Here's how the part is built. I have some questions about the finished solid (model axes, mm). A direction names the side the tool comes from. Round coordinates to 2 decimals unless told otherwise and drop trailing zeros. Order: outer loops, then holes, each group sorted by start corner. A loop starts at its lowest first (then second) coordinate and runs counter-clockwise, first axis right, second up. Notation, with made-up numbers: M -3,-17.5 L 41,-17.5 A18 cw 41,2.5 Z; hole C -7.75,19 d10. An arc over 180 degrees is marked long. Answer as CSV lines item,"result". Start each with the question number.
```python
from build123d import *
from build123d.topology import SkipClean

# Parameters (mm, degrees)
SKETCH1_W           = 25.4
SKETCH1_H           = 25.4
SKETCH1_R           = 1.5
BOSS_EXTRUDE1_DEPTH = 2.54
SKETCH3_W           = 25.4
SKETCH3_H           = 12.7
CUT_EXTRUDE1_DEPTH  = 19.139228208
BOSS_EXTRUDE2_START = 6.35
SKETCH4_R           = 3.175
SKETCH4_R_2         = 1.5
BOSS_EXTRUDE2_DEPTH = 6.35
FILLET1_R           = 6.35


with BuildPart() as part:
    # Sketch1 → Boss-Extrude1 (new body)
    with BuildSketch(Plane(origin=(0, 0, 0), x_dir=(1, 0, 0), z_dir=(0, 1, 0))):
        Rectangle(SKETCH1_W, SKETCH1_H)
        with Locations(Location((-6.35, 6.35, 0), (0, 0, 270))):
            Circle(SKETCH1_R, mode=Mode.SUBTRACT)
        with Locations(Location((6.35, 6.35, 0), (0, 0, 270))):
            Circle(SKETCH1_R, mode=Mode.SUBTRACT)
        with Locations(Location((6.35, -6.35, 0), (0, 0, 270))):
            Circle(SKETCH1_R, mode=Mode.SUBTRACT)
        with Locations(Location((-6.35, -6.35, 0), (0, 0, 270))):
            Circle(SKETCH1_R, mode=Mode.SUBTRACT)
    extrude(amount=BOSS_EXTRUDE1_DEPTH)

    # Sketch3 → Cut-Extrude1 (cut, through all)
    with BuildSketch(Plane.XZ):
        with Locations((0, -6.35)):
            Rectangle(SKETCH3_W, SKETCH3_H)
    extrude(amount=-CUT_EXTRUDE1_DEPTH, mode=Mode.SUBTRACT)

    # Sketch4 → Boss-Extrude2 (add)
    # profile 1 of 2: a face of its own
    with SkipClean():  # the faces are left unmerged after this step: merging them gives an invalid solid
        with BuildSketch(Plane.XZ.offset(BOSS_EXTRUDE2_START)):
            with Locations(Location((-6.35, 6.35, 0), (0, 0, 90))):
                Circle(SKETCH4_R)
            with Locations(Location((-6.35, 6.35, 0), (0, 0, 270))):
                Circle(SKETCH4_R_2, mode=Mode.SUBTRACT)
        # profile 2 of 2: a face of its own
        with BuildSketch(Plane.XZ.offset(BOSS_EXTRUDE2_START)):
            with Locations(Location((6.35, 6.35, 0), (0, 0, 90))):
                Circle(SKETCH4_R)
            with Locations(Location((6.35, 6.35, 0), (0, 0, 270))):
                Circle(SKETCH4_R_2, mode=Mode.SUBTRACT)
        extrude(amount=-BOSS_EXTRUDE2_DEPTH)

    # Fillet1
    fillet1_edges = [part.edges().sort_by_distance(p)[0] for p in [
        (12.7, 1.27, 0),
        (-12.7, 1.27, 0),
        (-12.7, 1.27, 12.7),
        (12.7, 1.27, 12.7),
    ]]
    fillet(fillet1_edges, radius=FILLET1_R - 0.0001)  # a hair under: the kernel refuses the full size

    # Fillet2: read off the stored shape, not the designer's step
    # Fillet2 outline → Fillet2 (revolve)
    with BuildSketch(Plane(origin=(6.35, 0, 6.35), x_dir=(1, 0, 0), z_dir=(0, 0, 1))):
        with BuildLine():
            ThreePointArc((3.175, -2.54), (3.918948776, -0.743948776), (5.715, 0))
            Line((5.715, 0), (3.175, 0))
            Line((3.175, 0), (3.175, -2.54))
        make_face()
    revolve(axis=Axis((6.35, 0, 6.35), (0, 1, 0)))

    # Fillet2 2 outline → Fillet2 2 (revolve)
    with BuildSketch(Plane(origin=(-6.35, 0, 6.35), x_dir=(1, 0, 0), z_dir=(0, 0, 1))):
        with BuildLine():
            ThreePointArc((3.175, -2.54), (3.918948776, -0.743948776), (5.715, 0))
            Line((5.715, 0), (3.175, 0))
            Line((3.175, 0), (3.175, -2.54))
        make_face()
    revolve(axis=Axis((-6.35, 0, 6.35), (0, 1, 0)))


solid = part.part
```
Item 1: For P1, Ø1, axis at x = 3.5, y = -4, coming from the +Z side (3 decimals); P2, Ø5, axis at x = -4.5, y = -4.5, coming from the +Z side (3 decimals); P3, Ø1, axis at y = 1.5, z = 7, coming from the -X side, each with a flat end and sliding along its axis, tell me the tip position at first contact or that it passes through.
Item 2: If we section it at D-D on y = -1.25: Please give me the cut outline in (x, z), and give its area (3 significant figures).
Item 3: Which directions (+Z, -Z, +X, -X, +Y, -Y) give clear straight access to the entire face, cutting with the end or side of a thin tool? Please do faces 4 (the cylindrical face through (-10.89, 1.29, 10.79)), 5 (the cylindrical face through (-3.25, -4.47, 5.66)).
Item 4: If I drill on line 1 along X through (y, z) = (-3, 6.35) (3 decimals); line 2 along X through (y, z) = (0.25, 6.35); line 3 along X through (y, z) = (1, 7.5), over which ranges is the centre line in solid material (lowest first)?
Item 5: If we section it at A-A on y = 1.25: Count the separate pieces of the cut face and the enclosed holes in it, and give its area (3 significant figures).
Item 6: If we section it at B-B on y = -4.5: Please give me the cut outline in (x, z) (3 decimals), and give its area (3 significant figures).
Item 7: We'd pull the mould along X, two halves only. Please class faces 1 (the cylindrical face through (10.79, 1.29, 1.81)), 2 (the flat face through (0, 1, 0)), 3 (the cylindrical face through (3.7, -4.5, 8.1)): pulls with the +X half, pulls with the -X half, needs draft (parallel to the pull), parting line crosses it, or undercut.
Geometry says:
1,P1,"z = 8.485"
1,P2,"z = 9.525"
1,P3,"x = -12.7"
2,outline,"C -6.35,6.35 d7.05; C 6.35,6.35 d7.05; hole C -6.35,6.35 d3; hole C 6.35,6.35 d3"
2,area,"64.0 mm²"
3,face 4,"+Z, -X, +Y, -Y"
3,face 5,"-Y"
4,line 1,"-9.525 to -7.85, -4.85 to -3.175, 3.175 to 4.85, 7.85 to 9.525"
4,line 2,"-12.7 to -7.85, -4.85 to 4.85, 7.85 to 12.7"
4,line 3,"-12.6 to -7.31, -5.39 to 5.39, 7.31 to 12.6"
5,separate pieces,"1"
5,enclosed holes,"2"
5,area,"274 mm²"
6,outline,"C -6.35,6.35 d6.35; C 6.35,6.35 d6.35; hole C -6.35,6.35 d3; hole C 6.35,6.35 d3"
6,area,"49.2 mm²"
7,face 1,"pulls with the +X half"
7,face 2,"needs draft"
7,face 3,"undercut"
